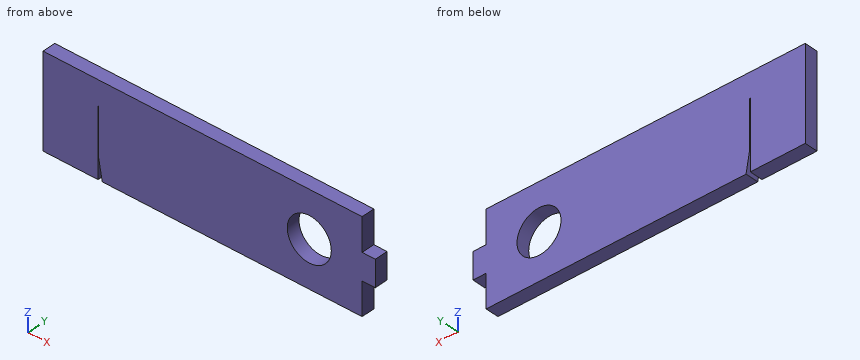
```python
from build123d import *

# Parameters (mm, degrees)
SKETCH1_W           = 145
SKETCH1_H           = 42
BOSS_EXTRUDE1_DEPTH = 6
SKETCH3_R           = 4
CUT_EXTRUDE1_DEPTH  = 7
SKETCH4_W           = 6
SKETCH4_H           = 12
BOSS_EXTRUDE2_DEPTH = 6
BOSS_EXTRUDE3_DEPTH = 6
SKETCH7_R           = 0.75
CUT_EXTRUDE2_DEPTH  = 7
CUT_EXTRUDE3_DEPTH  = 7
SKETCH9_R           = 10
CUT_EXTRUDE4_DEPTH  = 10


with BuildPart() as part:
    # Sketch1 → Boss-Extrude1 (new body)
    with BuildSketch(Plane(origin=(0, 0, 0), x_dir=(1, 0, 0), z_dir=(0, 1, 0))):
        Rectangle(SKETCH1_W, SKETCH1_H)
    extrude(amount=BOSS_EXTRUDE1_DEPTH)

    # Sketch3 → Cut-Extrude1 (cut, through all)
    with BuildSketch(Plane.XZ):
        with Locations((48.5, 0)):
            Circle(SKETCH3_R)
    extrude(amount=-CUT_EXTRUDE1_DEPTH, mode=Mode.SUBTRACT)

    # Sketch4 → Boss-Extrude2 (add)
    with BuildSketch(Plane(origin=(0, 6, 0), x_dir=(1, 0, 0), z_dir=(0, 1, 0))):
        with Locations((75.5, 0)):
            Rectangle(SKETCH4_W, SKETCH4_H)
    extrude(amount=-BOSS_EXTRUDE2_DEPTH)

    # Sketch5 → Boss-Extrude3 (add)
    with BuildSketch(Plane(origin=(0, 6, 0), x_dir=(1, 0, 0), z_dir=(0, 1, 0))):
        Polygon((-59.5, -10), (-72.5, -10), (-72.5, -21), (-53.5, -21), (-53.5, -17.5), (-59.5, -17.5), align=None)
    extrude(amount=-BOSS_EXTRUDE3_DEPTH)

    # Sketch7 → Cut-Extrude2 (cut, through all)
    with BuildSketch(Plane.XZ):
        with Locations((-161.479103552, -154.351327649)):
            Circle(SKETCH7_R)
    extrude(amount=-CUT_EXTRUDE2_DEPTH, mode=Mode.SUBTRACT)

    # Sketch8 → Cut-Extrude3 (cut, through all)
    with BuildSketch(Plane(origin=(0, 6, 0), x_dir=(1, 0, 0), z_dir=(0, 1, 0))):
        Polygon((-47.5, 21), (-47.5, -10), (-47.2, -10), (-47.2, 11.701384546), (-45.560403212, 21), align=None)
    extrude(amount=-CUT_EXTRUDE3_DEPTH, mode=Mode.SUBTRACT)

    # Sketch9 → Cut-Extrude4 (cut)
    with BuildSketch(Plane(origin=(0, 6, 0), x_dir=(1, 0, 0), z_dir=(0, 1, 0))):
        with Locations((48.5, 0)):
            Circle(SKETCH9_R)
    extrude(amount=-CUT_EXTRUDE4_DEPTH, mode=Mode.SUBTRACT)


solid = part.part
```
Geometry: final body of the model. Coordinates: model frame, mm. Round coordinates to 2 decimals unless told otherwise and drop trailing zeros. Write each loop counter-clockwise with the first axis right and the second up, starting at its lowest first coordinate (ties: lowest second). Pieces come first, ordered by that corner, then holes. Notation, with made-up numbers: (44.5, -0.75) -> (66.5, -0.75) arc R25 cw to (66.5, 21.25) -> close; hole circle Ø7 at (-3, 37). An arc over 180 degrees is marked (long way). Return JSON: item names as keys, results as strings.
Q1. Section A-A on y = 4.5. Return the cut outline in (x, z), and give its area (3 significant figures).
From the geometry:
{"outline": "(-72.5, -21) -> (-47.5, -21) -> (-47.5, 10) -> (-47.2, 10) -> (-47.2, -11.7) -> (-45.56, -21) -> (72.5, -21) -> (72.5, -6) -> (78.5, -6) -> (78.5, 6) -> (72.5, 6) -> (72.5, 21) -> (-72.5, 21) -> close; hole circle Ø20 at (48.5, 0)", "area": "5,830 mm2"}
Q2. First-contact query: pin 1 Ø3 at (x, y) = (74.5, 3.5) entering from -Z; pin 2 Ø1.8 at (y, z) = (2, 11.5) entering from +X. Flat tips, straight axial feed; report the tip coordinate or a pass-through.
From the geometry:
{"pin 1": "z = -6", "pin 2": "x = 72.5"}
Q3. Section C-C on x = 48.5. Return the cut outline in (y, z), and give its area (3 significant figures).
From the geometry:
{"outline": "(0, -21) -> (6, -21) -> (6, -10) -> (0, -10) -> close; (0, 10) -> (6, 10) -> (6, 21) -> (0, 21) -> close", "area": "132 mm2"}
Q4. Section B-B on z = 0. Return the cut outline in (x, y), and give its area (3 significant figures).
From the geometry:
{"outline": "(-72.5, 0) -> (-47.5, 0) -> (-47.5, 6) -> (-72.5, 6) -> close; (-47.2, 0) -> (38.5, 0) -> (38.5, 6) -> (-47.2, 6) -> close; (58.5, 0) -> (78.5, 0) -> (78.5, 6) -> (58.5, 6) -> close", "area": "784 mm2"}
Q5. Ray query, line 1 (X direction, y = 2.3, z = 0); line 2 (X direction, y = 3, z = 3); line 3 (Z direction, x = 48.5, y = 1.55). Return the intervals inside material, ascending.
From the geometry:
{"line 1": "-72.5 to -47.5, -47.2 to 38.5, 58.5 to 78.5", "line 2": "-72.5 to -47.5, -47.2 to 38.96, 58.04 to 78.5", "line 3": "-21 to -10, 10 to 21"}
